Geometry check sheet. Reference: the model listing, model coordinates, mm. A direction names the side the tool comes from. Give positions to 0.01 mm unless a question says otherwise; leave off trailing zeros. Write each loop counter-clockwise with the first axis right and the second up, starting at its lowest first coordinate (ties: lowest second). Pieces come first, ordered by that corner, then holes. Notation, with made-up numbers: (76.25, 10.25) -> (110.25, 10.25) arc R28 cw to (110.25, 38.25) -> close; hole circle Ø8 at (-38, 59). An arc over 180 degrees is marked (long way). One line per item, written item: value.
Autodesk Inventor part; units mm, degrees
ref_plane "YZ Plane" through (0, 0, 0) normal (1, 0, 0) x (0, 1, 0)
ref_plane "XZ Plane" through (0, 0, 0) normal (0, 1, 0) x (-1, 0, 0)
ref_plane "XY Plane" through (0, 0, 0) normal (0, 0, 1) x (1, 0, 0)
sketch "스케치1" plane through (0, 0, 0) normal (0, 1, 0) x (-1, 0, 0)
  line L0 (65, -14) -> (-65, -14)
  line L1 (-65, -14) -> (-65, 14)
  line L2 (-65, 14) -> (65, 14)
  line L3 (65, 14) -> (65, -14)
  point P0 (0, 0)
  dimension "d0" = 28
  dimension "d1" = 130
  dimension "d2" = 14
  dimension "d3" = 65
extrude "돌출1" add sketch "스케치1" along normal blind 7
sketch "스케치4" plane through (0, 0, 0) normal (0, -1, 0) x (1, 0, 0)
  line L0 (-65, -14) -> (65, -14)
  line L1 (65, 14) -> (-65, 14)
  line L2 (-65, -14) -> (-57, -14)
  line L3 (-57, -14) -> (-57, 14)
  line L4 (-57, 14) -> (-65, 14)
  line L5 (-65, 14) -> (-65, -14)
  point P0 (0, 0)
  point P1 (63, -14)
  point P2 (63, 14)
  dimension "d26" = 8
extrude "돌출4" add sketch "스케치4" along normal blind 124
fillet "모깎기2" radius 2 1 edges at (-65, 7, 0)
sketch "스케치5" plane through (-57, 0, 14) normal (1, 0, 0) x (0, 0, -1)
  point P0 (14, 0)
sketch "스케치10" plane through (-57, 0, 14) normal (1, 0, 0) x (0, 0, -1)
  line L0 (0, -124) -> (28, -124)
  line L1 (28, -124) -> (28, 5)
  line L2 (0, -124) -> (28, -124)
  line L3 (28, -124) -> (28, -117)
  line L4 (28, -117) -> (0, -117)
  line L5 (0, -117) -> (0, -124)
  point P0 (14, 0)
  dimension "d52" = 7
extrude "돌출9" add sketch "스케치10" along normal blind 122
sketch "스케치2" plane through (0, 7, 0) normal (0, 1, 0) x (1, 0, 0)
  circle A0 centre (61, 0) radius 5
  line L0 (61, 5) -> (65, 5)
  line L1 (65, 5) -> (65, -5)
  line L2 (65, -5) -> (61, -5)
  line L3 (61, -5) -> (61, 5)
  line L4 (65, -14) -> (65, 14)
  point P0 (0, 0)
  dimension "d6" = 10
  dimension "d7" = 0
  dimension "d8" = 10
  dimension "d9" = 5
  dimension "d10" = 4
  dimension "d11" = 0
extrude "돌출2" cut sketch "스케치2" against normal blind 180
sketch "스케치3" plane through (0, 7, 0) normal (0, 1, 0) x (1, 0, 0)
  circle A0 centre (62, 11) radius 1.25
  line L0 (65, 5) -> (65, 14)
  line L1 (65, 14) -> (-65, 14)
  line L2 (0, 0) -> (4.9885, 0)
  circle A1 centre (62, -11) radius 1.25
  circle A2 centre (51, 0) radius 1.25
  line L3 (-65, -14) -> (65, -14)
  circle A3 centre (54.222, -7.778) radius 1.25
  line L4 (65, -14) -> (65, -5)
  circle A4 centre (54.222, 7.778) radius 1.25
  dimension "d14" = 2.5
  dimension "d15" = 3
  dimension "d16" = 3
  dimension "d17" = 14
  dimension "d18" = 2.5
  dimension "d19" = 14
  dimension "d20" = 10.778
  dimension "d21" = 6.222
  dimension "d22" = 2.5
extrude "돌출3" cut sketch "스케치3" against normal blind 100000
fillet "모깎기4" radius 2 5 edges at (65, -120.5, 14) (65, -120.5, -14) (65, 3.5, -14) (65, 3.5, 14) (-65, -124, 0)
sketch "스케치11" plane through (-57, -117, 14) normal (0, 0, 1) x (1, 0, 0)
  circle A0 centre (-6, 47.5) radius 1.5
  circle A1 centre (-6, 69.5) radius 1.5
  line L0 (-8, 122) -> (-8, -5)
  line L1 (181.1056, 58.5) -> (-67.096, 58.5)
  point P0 (57, 117)
  dimension "d56" = 3
  dimension "d57" = 3
  dimension "d58" = 2
  dimension "d59" = 2
  dimension "d60" = 22
  dimension "d61" = 58.5
  dimension "d62" = 11
extrude "돌출10" cut sketch "스케치11" against normal blind 122
sketch "스케치12" plane through (-57, 0, 14) normal (1, 0, 0) x (0, 0, -1)
  line L0 (7, -33.5) -> (21, -33.5)
  line L1 (21, -33.5) -> (21, -83.5)
  line L2 (21, -83.5) -> (7, -83.5)
  line L3 (7, -83.5) -> (7, -33.5)
  line L4 (0, 0) -> (0, -117)
  line L5 (28, 0) -> (28, -117)
  line L6 (-36.3144, -58.5) -> (56.0369, -58.5)
  line L7 (9, -117) -> (19, -117)
  point P0 (14, 0)
  dimension "d65" = 7
  dimension "d66" = 7
  dimension "d67" = 50
  dimension "d68" = 58.5
  dimension "d69" = 25
extrude "돌출11" cut sketch "스케치12" against normal blind 122
sketch "스케치13" plane through (0, -124, 0) normal (0, -1, 0) x (1, 0, 0)
  line L0 (-63, 14) -> (63, 14)
  line L1 (47, 14) -> (65, 14)
  line L2 (65, 14) -> (65, -15.4156)
  line L3 (65, -15.4156) -> (47, -15.4156)
  line L4 (47, -15.4156) -> (47, 14)
  line L5 (65, 12) -> (65, 5)
  point P0 (0, 0)
  dimension "d72" = 18
  dimension "d73" = 0
extrude "돌출12" cut sketch "스케치13" against normal blind 3
sketch "스케치14" plane through (0, 7, 0) normal (0, 1, 0) x (1, 0, 0)
  line L0 (-57, -14) -> (63, -14)
  line L1 (-57, 14) -> (63, 14)
  line L2 (47, -14) -> (65, -14)
  line L3 (65, -14) -> (65, 14)
  line L4 (65, 14) -> (47, 14)
  line L5 (47, 14) -> (47, -14)
  line L6 (65, -12) -> (65, -5)
  point P0 (0, 0)
  dimension "d76" = 18
  dimension "d77" = 0
extrude "돌출13" cut sketch "스케치14" against normal blind 3
chamfer "모따기1" distance 3 angle 45 2 edges at (47, 7, 0) (47, -124, 0)
properties part number "shoulder_gear_3"
1) Scan lines: probe 1 along Z at (x, y) = (62, -118.1); probe 2 along Y at (x, z) = (-13, 11.75); probe 3 along Y at (x, z) = (47.5, 3.5). Record each from-to range of solid material in increasing order.
Verdict:
probe 1: -14 to -12.25, -9.75 to -5, 5 to 9.75, 12.25 to 14
probe 2: -124 to -117, 0 to 7
probe 3: -121 to -117, 0 to 4
2) Tool access check on faces 5 (the flat face through (63, -119, -5)), 6 (the flat face through (54, 4, 0)), 7 (the flat face through (-57, -58, -10)), 8 (the flat face through (54, -121, 0)), 9 (the flat face through (-61, -58, -7)). Record the directions out of +Z, -Z, +X, -X, +Y, -Y that give a thin tool (end or side, any length) a straight path to the whole face; none if there is none.
Verdict:
face 5: +X, +Y, -Y
face 6: +Z, -Z, +X, +Y
face 7: +Z, -Z, +X
face 8: +Z, -Z, +X, -Y
face 9: +X, -X
3) Mould release check, pull along Z, two halves, no side actions. Record for faces 1 (the flat face through (-61, -33.5, 0)), 2 (the flat face through (-58, -73, -14)), 3 (the flat face through (-58, -44, 14)), 4 (the flat face through (65, -119, -8)): released by +Z, released by -Z, zero draft, split by the parting line, or undercut.
Verdict:
face 1: undercut
face 2: released by -Z
face 3: released by +Z
face 4: zero draft
4) Sectioned sample at D-D on y = -6. Record the cut outline in (x, z), plus the area to 3 significant figures.
Verdict:
outline: (-65, -14) -> (-57, -14) -> (-57, 14) -> (-65, 14) -> close
area: 224 mm^2
5) Sectioned sample at C-C on y = -69.5. Record the cut outline in (x, z).
Verdict:
outline: (-65, -14) -> (-64.5, -14) -> (-64.5, -7) -> (-65, -7) -> close; (-65, 7) -> (-64.5, 7) -> (-64.5, 14) -> (-65, 14) -> close; (-61.5, -14) -> (-57, -14) -> (-57, -7) -> (-61.5, -7) -> close; (-61.5, 7) -> (-57, 7) -> (-57, 14) -> (-61.5, 14) -> close
6) Sectioned sample at B-B on x = 19. Record the cut outline in (y, z).
Verdict:
outline: (-124, -14) -> (-117, -14) -> (-117, 14) -> (-124, 14) -> close; (0, -14) -> (7, -14) -> (7, 14) -> (0, 14) -> close
7) Depth check by flat-ended pin: pin 1 Ø4 at (x, z) = (51, 0) entering from +Y; pin 2 Ø2 at (x, z) = (54.222, 7.778) entering from +Y; pin 3 Ø1 at (y, z) = (-74, -9.5) entering from +X; pin 4 Ø3 at (x, z) = (62, -11) entering from -Y. Enter the tip coordinate at first touch or a pass-through.
Verdict:
pin 1: y = 4
pin 2: through
pin 3: x = -57
pin 4: y = -121
